Geometry: see drawing. Coordinates: mm, zero at the bounding-box minimum. Coordinates: 2 decimals unless noted, no trailing zeros. Loops run counter-clockwise (first coordinate to the right, second up) from the corner with the lowest first, then second, coordinate; pieces in that order, holes last. Notation, with made-up numbers: (-13, 71.5) -> (-8, 71.5) arc R12 cw to (-8, 92.5) -> close; hole circle Ø8 at (46.25, -9). An arc over 180 degrees is marked (long way). One line per item, written item: value. Start each with the question number.
Item 1: Ray query, probe 1 along X at (y, z) = (65, 3.25); probe 2 along Y at (x, z) = (35.5, 1); probe 3 along Y at (x, z) = (54, 6). Return the intervals inside material, ascending. Write a range as from..to.
Item 2: Section query A-A on y = 74. Return loops of the section in (x, z).
Item 3: Contact query for a flat-ended pin moving along its axis: pin 1 Ø5 at (x, y) = (65.5, 119) entering from -Z. Output: stop coordinate, or through.
Item 4: Section query B-B on x = 30. Return loops of the section in (y, z).
Item 5: Section query C-C on z = 5.25. Return loops of the section in (x, y) (3 decimals).
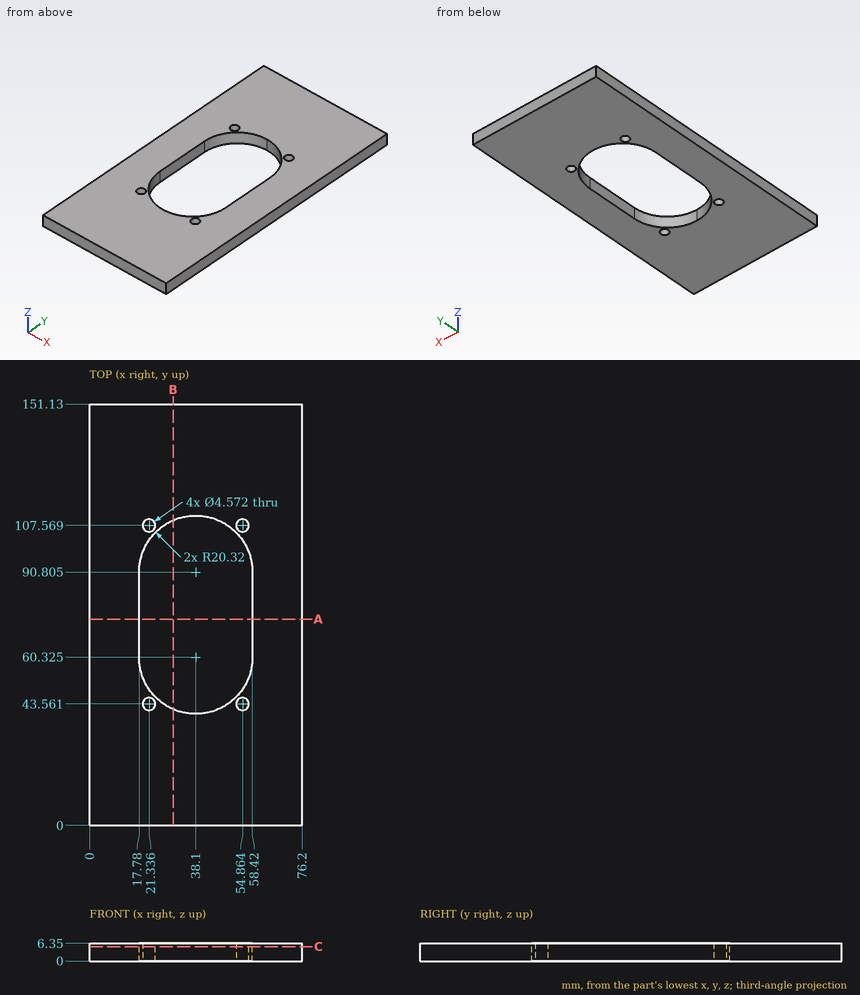
Reply:
1. probe 1: x = 0..17.78, 58.42..76.2
1. probe 2: y = 0..40.17, 110.96..151.13
1. probe 3: y = 0..41.44, 45.68..47.67, 103.46..105.45, 109.69..151.13
2. outline: (0, 0) -> (17.78, 0) -> (17.78, 6.35) -> (0, 6.35) -> close; (58.42, 0) -> (76.2, 0) -> (76.2, 6.35) -> (58.42, 6.35) -> close
3. pin 1: stops at z = 0
4. outline: (0, 0) -> (41.69, 0) -> (41.69, 6.35) -> (0, 6.35) -> close; (109.44, 0) -> (151.13, 0) -> (151.13, 6.35) -> (109.44, 6.35) -> close
5. outline: (0, 0) -> (76.2, 0) -> (76.2, 151.13) -> (0, 151.13) -> close; hole (17.78, 60.325) arc R20.32 ccw to (38.1, 40.005) arc R20.32 ccw to (58.42, 60.325) -> (58.42, 90.805) arc R20.32 ccw to (38.1, 111.125) arc R20.32 ccw to (17.78, 90.805) -> close; hole circle Ø4.572 at (21.336, 43.561); hole circle Ø4.572 at (21.336, 107.569); hole circle Ø4.572 at (54.864, 43.561); hole circle Ø4.572 at (54.864, 107.569)
